Design review of the part built by this model. Coordinates are the model's own, in mm. A direction names the side the tool comes from. Give positions to 0.01 mm unless a question says otherwise; leave off trailing zeros. Loops run counter-clockwise (first coordinate to the right, second up) from the corner with the lowest first, then second, coordinate; pieces in that order, holes last. Notation, with made-up numbers: (-15, 39.25) - (11, 39.25) arc R22 ccw to (11, 72.25) - close; hole circle Ø2 at (60.25, 19.25). An arc over 180 degrees is marked (long way). Write each question's results on one line, items separated by ' | '.
```python
from build123d import *

# Parameters (mm, degrees)
ENL_V_MAT_EXTRU_1_DEPTH = 1.2
CHANFREIN1_SIZE         = 0.15


with BuildPart() as part:
    # Esquisse1 → Révolution1 (revolve)
    with BuildSketch(Plane.XY, mode=Mode.PRIVATE) as r_volution1_sk:
        with BuildLine():
            Line((1, -7.6), (0.6, -8))
            Line((0.6, -8), (0, -8))
            Line((0, -8), (0, 2))
            Line((0, 2), (1.5, 2))
            ThreePointArc((1.5, 2), (1.782842712, 1.882842712), (1.9, 1.6))
            Line((1.9, 1.6), (1.9, 0))
            Line((1.9, 0), (1, 0))
            Line((1, 0), (1, -7.6))
        make_face()
    revolve(r_volution1_sk.sketch.rotate(Axis((0, 6.972972973, 0), (0, -1, 0)), 90), axis=Axis((0, 6.972972973, 0), (0, -1, 0)))

    # Esquisse2 → Enlèv. mat.-Extru.1 (cut)
    with BuildSketch(Plane(origin=(0, 2, 0), x_dir=(1, 0, 0), z_dir=(0, 1, 0))):
        Polygon((-0.866025404, 0), (-0.433012702, -0.75), (0.433012702, -0.75), (0.866025404, 0), (0.433012702, 0.75), (-0.433012702, 0.75), align=None)
    extrude(amount=-ENL_V_MAT_EXTRU_1_DEPTH, mode=Mode.SUBTRACT)

    # Chanfrein1
    chanfrein1_edges = [part.edges().sort_by_distance(p)[0] for p in [
        (-0.649519053, 2, -0.375),
        (-0.649519053, 2, 0.375),
        (0, 2, 0.75),
        (0.649519053, 2, 0.375),
        (0.649519053, 2, -0.375),
        (0, 2, -0.75),
    ]]
    chamfer(chanfrein1_edges, length=CHANFREIN1_SIZE)


solid = part.part
```
Item 1: Tool access review of faces 4 (the face through (0, 1, -0.75)), 5 (the face through (1, -4, 0)), 6 (the face through (0, -8, 0)): name each direction out of +Z, -Z, +X, -X, +Y, -Y from which nothing blocks a thin tool from reaching the whole face with its end or side.
Output values:
face 4: +Y | face 5: -Y | face 6: +Z, -Z, +X, -X, -Y
Item 2: Clearance check with a flat-ended pin moving along its axis: P1, Ø0.8, axis at x = 0, z = 0, coming from the +Y side. State where the tip first meets the part, or that it passes through.
Output values:
P1: stops at y = 0.8
Item 3: Draft analysis for pull direction X (two halves, no side actions). For faces 1 (the face through (0, 1, 0.75)), 2 (the face through (1, 0, 1)), 3 (the face through (-0.571, 0.789, 1.812)), state which applies: +X half, -X half, draft (parallel to the pull), parting line (faces both ways), or undercut.
Output values:
face 1: undercut | face 2: draft | face 3: parting line
Item 4: We need section C-C on y = -4.75. Give the boundary of the cut face in (x, z).
Output values:
outline: circle Ø2 at (0, 0)
Item 5: We need section A-A on y = 1. Give the boundary of the cut face in (x, z).
Output values:
outline: circle Ø3.8 at (0, 0); hole (-0.87, 0) - (-0.43, -0.75) - (0.43, -0.75) - (0.87, 0) - (0.43, 0.75) - (-0.43, 0.75) - close
Item 6: We need section B-B on x = 0. Give the boundary of the cut face in (y, z), then the cut area to 3 significant figures.
Output values:
outline: (-8, -0.6) - (-7.6, -1) - (0, -1) - (0, -1.9) - (1.6, -1.9) arc R0.4 ccw to (2, -1.5) - (2, -0.9) - (1.85, -0.75) - (0.8, -0.75) - (0.8, 0.75) - (1.85, 0.75) - (2, 0.9) - (2, 1.5) arc R0.4 ccw to (1.6, 1.9) - (0, 1.9) - (0, 1) - (-7.6, 1) - (-8, 0.6) - close | area: 21.5 mm²
Item 7: Wall thickness on probe 1 along Y at (x, z) = (0.5, 1.1); probe 2 along Y at (x, z) = (-0.5, 0.2); probe 3 along X at (y, z) = (-6, 0.7): over which ranges is each line inside the solid? List them lowest first.
Output values:
probe 1: y = 0 to 2 | probe 2: y = -8 to 0.8 | probe 3: x = -0.71 to 0.71
